The model under review builds one solid part; all positions refer to its coordinate system, in mm. A direction names the side the tool comes from. Coordinates: 2 decimals unless noted, no trailing zeros. Write each loop counter-clockwise with the first axis right and the second up, starting at its lowest first coordinate (ties: lowest second). Pieces come first, ordered by that corner, then holes. Notation, with made-up numbers: (32, 7) - (73, 7) arc R24 cw to (73, 32) - close; hole circle Ø6 at (-32.75, 83.25). An arc over 180 degrees is marked (long way). Use one line per item in the form item = value. Start each with the question number.
```python
from build123d import *

# Parameters (mm, degrees)
SKETCH1_R           = 14
SKETCH1_R_2         = 9
BOSS_EXTRUDE1_DEPTH = 35
SKETCH3_R           = 8.950574332
BOSS_EXTRUDE2_DEPTH = 9.5
BOSS_EXTRUDE3_DEPTH = 2.5
SKETCH7_W           = 5
SKETCH7_H           = 35
BOSS_EXTRUDE5_DEPTH = 0.225023
RIB12_REACH         = 63.664
SKETCH6_WALL_W      = 163.51256394
SKETCH6_WALL_H      = 10


with BuildPart() as part:
    # Sketch1 → Boss-Extrude1 (new body)
    with BuildSketch(Plane.XY):
        Circle(SKETCH1_R)
        Circle(SKETCH1_R_2, mode=Mode.SUBTRACT)
    extrude(amount=BOSS_EXTRUDE1_DEPTH)



with BuildPart() as body_2:
    # Sketch3 → Boss-Extrude2 (new, symmetric)
    with BuildSketch(Plane(origin=(0, 0, 0), x_dir=(0, 0, -1), z_dir=(1, 0, 0))):
        with Locations((-17.5, 48.496368985)):
            Circle(SKETCH3_R)
    extrude(amount=BOSS_EXTRUDE2_DEPTH, both=True)

    # Sketch3<3> → Boss-Extrude3 (add, symmetric)
    with BuildSketch(Plane(origin=(0, 0, 0), x_dir=(0, 0, -1), z_dir=(1, 0, 0))):
        with BuildLine():
            Line((-26.202553454, 50.588818327), (-35, 14))
            Line((-35, 14), (0, 14))
            Line((0, 14), (-8.797446546, 50.588818327))
            ThreePointArc((-8.797446546, 50.588818327), (-8.61164716, 49.549917585), (-8.549425668, 48.496368985))
            ThreePointArc((-8.549425668, 48.496368985), (-18.553548599, 39.608016145), (-26.202553454, 50.588818327))
        make_face()
    extrude(amount=BOSS_EXTRUDE3_DEPTH, both=True)


with BuildPart() as part_1:
    add(part.part)

    add(body_2.part)  # Boss-Extrude5 merges body 2
    # Sketch7 → Boss-Extrude5 (add)
    with BuildSketch(Plane.XZ.offset(-14)):
        with Locations((0, 17.5)):
            Rectangle(SKETCH7_W, SKETCH7_H)
    extrude(amount=BOSS_EXTRUDE5_DEPTH)

    # Sketch6 wall → Rib12 (add, up to next)
    with BuildSketch(Plane(origin=(11.703236177, 20.580676171, 17.5), x_dir=(0.115396977809, -0.993319453908, 0), z_dir=(-0.993319453908, -0.115396977809, 0)), mode=Mode.PRIVATE) as rib12_sk1:
        Rectangle(SKETCH6_WALL_W, SKETCH6_WALL_H)
    rib12_tool1 = extrude(rib12_sk1.sketch, amount=RIB12_REACH, mode=Mode.PRIVATE) - part_1.part
    rib12 = rib12_tool1.solids().sort_by_distance((11.703236177, 20.580676171, 17.5))[0]
    add(rib12)

    # Mirror1: Rib12 across plane
    add(rib12.mirror(Plane(origin=(0, 0, 0), x_dir=(0, 0, 1), z_dir=(1, 0, 0))))


solid = part_1.part
```
1. Take a section at B-B (x = 0). State the section outline as (y, z) points, plus the area to 3 significant figures.
2. Take a section at A-A (y = 0). State the section outline as (x, z) points, plus the area to 3 significant figures.
3. The part is to be moulded in two halves that separate along Y. For faces 5 (the flat face through (3, -9, 35)), 6 (the flat face through (7, 26, 12.5)), 7 (the flat face through (0.035, 32.038, 4.337)), say which applies: released by +Y, released by -Y, zero draft, split by the parting line, or undercut.
4. For P1, Ø10, axis at y = 27, z = 29, coming from the +X side; P2, Ø12, axis at y = 22.5, z = 25.5, coming from the -X side; P3, Ø6, axis at x = -7, z = 10.5, coming from the -Y side; P4, Ø6, axis at x = -3.5, y = -4, coming from the -Z side, all flat-tipped, find the tip position at first contact; note any pin that passes through.
5. Take a section at D-D (x = 10.5). State the section outline as (y, z) points.
6. For L1, parallel to X at y = 26.5, z = 9; L2, parallel to Z at x = 9.75, y = 15.5; L3, parallel to Y at x = 3.5, z = 19, list the stretches that pass through material, from the lowest coordinate up.
7. For faces 1 (the flat face through (2.5, 28, 8)), 2 (the cylindrical face through (-0.58, -13.988, 17.255)), 3 (the flat face through (-2.5, 28, 8)), 4 (the flat face through (7, 26, 22.5)), list the 3-axis set-ups (+Z, -Z, +X, -X, +Y, -Y) from which the entire face can be reached by the end or side of a thin tool; tool diameter is ignored.
Returned:
q1.outline = (-14, 0) - (-9, 0) - (-9, 35) - (-14, 35) - close; (9, 0) - (14, 0) - (50.59, 8.8) arc R8.95 ccw to (50.59, 26.2) - (14, 35) - (9, 35) - close
q1.area = 1,400 mm²
q2.outline = (-14, 0) - (-9, 0) - (-9, 35) - (-14, 35) - close; (9, 0) - (14, 0) - (14, 35) - (9, 35) - close
q2.area = 350 mm²
q3.face_5 = zero draft
q3.face_6 = undercut
q3.face_7 = released by +Y
q4.P1 = 2.5
q4.P2 = -12.08
q4.P3 = -13.42
q4.P4 = through
q5.outline = (-9.26, 0) - (9.26, 0) - (9.26, 12.5) - (30.94, 12.5) - (30.94, 22.5) - (9.26, 22.5) - (9.26, 35) - (-9.26, 35) - close
q6.L1 = -2.5 to 2.5
q6.L2 = 12.5 to 22.5
q6.L3 = -13.56 to -8.29, 8.29 to 57.32
q7.face_1 = -Z, +X
q7.face_2 = none
q7.face_3 = -Z, -X
q7.face_4 = +Z, +X
